Here's how the part is built. I have some questions about the finished solid (model axes, mm). Face numbers are marked on the shaded views. A direction names the side the tool comes from. Give positions to 0.01 mm unless a question says otherwise; leave off trailing zeros. Order: outer loops, then holes, each group sorted by start corner. A loop starts at its lowest first (then second) coordinate and runs counter-clockwise, first axis right, second up.
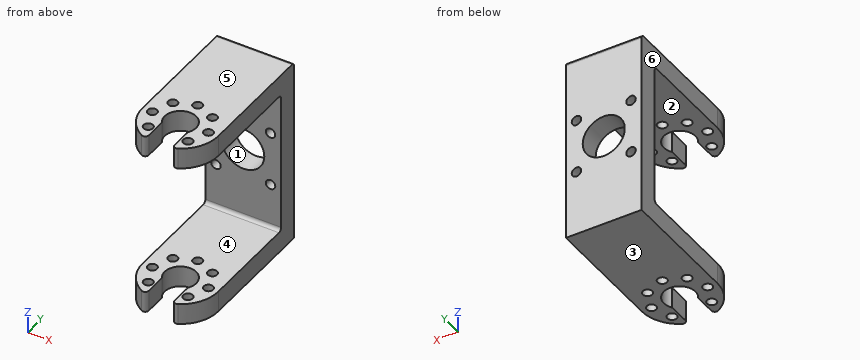
Autodesk Inventor part; units mm, degrees
ref_plane "YZ Plane" through (0, 0, 0) normal (1, 0, 0) x (0, 1, 0)
ref_plane "XZ Plane" through (0, 0, 0) normal (0, 1, 0) x (-1, 0, 0)
ref_plane "XY Plane" through (0, 0, 0) normal (0, 0, 1) x (1, 0, 0)
sketch "스케치1" plane through (0, 0, 0) normal (0, 0, 1) x (1, 0, 0)
  circle A0 centre (-22.9272, 17.0843) radius 10.8
  circle A1 centre (-22.9272, 17.0843) radius 6
  circle A2 centre (-22.9272, 9.0843) radius 1.05
  circle A3 centre (-28.584, 11.4274) radius 1.05
  circle A4 centre (-30.9272, 17.0843) radius 1.05
  circle A5 centre (-28.584, 22.7411) radius 1.05
  circle A6 centre (-22.9272, 25.0843) radius 1.05
  circle A7 centre (-17.2703, 22.7411) radius 1.05
  circle A8 centre (-14.9272, 17.0843) radius 1.05
  circle A9 centre (-17.2703, 11.4274) radius 1.05
  circle A10 centre (-28.584, 22.7411) radius 1.15
  circle A11 centre (-22.9272, 25.0843) radius 1.15
  circle A12 centre (-17.2703, 22.7411) radius 1.15
  circle A13 centre (-14.9272, 17.0843) radius 1.15
  circle A14 centre (-17.2703, 11.4274) radius 1.15
  circle A15 centre (-28.584, 11.4274) radius 1.15
  circle A16 centre (-30.9272, 17.0843) radius 1.15
  circle A17 centre (-22.9272, 17.0843) radius 3.5
  arc A18 (-19.2272, 17.0843) -> (-26.6272, 17.0843) centre (-22.9272, 17.0843) ccw
  arc A19 (-19.2272, 6.9378) -> (-26.6272, 6.9378) centre (-22.9272, 17.0843) ccw
  line L0 (-26.6272, 17.0843) -> (-26.6272, 6.9378)
  line L1 (-19.2272, 17.0843) -> (-19.2272, 6.9378)
  line L2 (-33.7272, 17.0843) -> (-33.7272, 52.0843)
  line L3 (-12.1272, 17.0843) -> (-12.1272, 52.0843)
  line L4 (-12.1272, 52.0843) -> (-33.7272, 52.0843)
  line L5 (-33.7272, 52.0843) -> (-12.1272, 52.0843)
  line L6 (-12.1272, 52.0843) -> (-12.1272, 58.0843)
  line L7 (-12.1272, 58.0843) -> (-33.7272, 58.0843)
  line L8 (-33.7272, 58.0843) -> (-33.7272, 52.0843)
  point P0 (0, 0)
  dimension "d0" = 0.1
  dimension "d1" = 0.1
  dimension "d2" = 0.1
  dimension "d3" = 0.1
  dimension "d4" = 0.1
  dimension "d5" = 0.1
  dimension "d6" = 0.1
  dimension "d7" = 0.2
  dimension "d8" = 35
  dimension "d9" = 35
  dimension "d10" = 6
extrude "돌출1" add sketch "스케치1" along normal blind 6 contours A0 L1 A1 L0 | A0 L2 L4 L3 | L1 A18 L0 A1 | A3 | A4 | A5 | A6 | A7 | A8 | A9 | A10 | A11 | A12 | A13 | A14 | A15 | A16 picked at (-19.6686, 25.2568) picked at (-26.9638, 14.2707)
sketch "스케치3" plane through (-33.7272, 52.0843, 0) normal (0, 1, 0) x (1, 0, 0)
  line L0 (0, -5.5) -> (21.6, -5.5)
  line L1 (21.6, -5.5) -> (21.6, 0.5)
  line L2 (0, -5.5) -> (0, 0.5)
  line L3 (0, -5.5) -> (21.6, -5.5)
  line L4 (0, -5.5) -> (21.6, -5.5)
  line L5 (21.6, -5.5) -> (21.6, 0.5)
  line L6 (0, -5.5) -> (0, 0.5)
  circle A0 centre (3.0218, -2.5) radius 1.45
  circle A1 centre (18.5782, -2.5) radius 1.45
  line L7 (21.6, 0.5) -> (21.6, 0)
  line L8 (21.6, 0) -> (0, 0)
  line L9 (0, 0) -> (0, 0.5)
  line L10 (21.6, 0) -> (0, 0)
  line L11 (0, 0) -> (0, -6)
  line L12 (21.6, -6) -> (0, -6)
  line L13 (21.6, 0) -> (21.6, -6)
  circle A2 centre (10.8, 20.55) radius 6
  line L14 (0, 0) -> (21.6, 0)
  line L15 (21.6, 0) -> (21.6, 41.1)
  line L16 (21.6, 41.1) -> (0, 41.1)
  line L17 (0, 41.1) -> (0, 0)
  line L18 (0, 41.1) -> (21.6, 41.1)
  line L19 (21.6, 41.1) -> (21.6, 47.1)
  line L20 (21.6, 47.1) -> (0, 47.1)
  line L21 (0, 47.1) -> (0, 41.1)
  circle A3 centre (18.5782, 12.7718) radius 1.35
  circle A4 centre (18.5782, 28.3282) radius 1.35
  circle A5 centre (3.0218, 28.3282) radius 1.35
  circle A6 centre (3.0218, 12.7718) radius 1.35
  point P0 (33.7272, 0)
  dimension "d13" = 2.9
  dimension "d14" = 2.9
  dimension "d19" = 0.5
  dimension "d24" = 12
  dimension "d25" = 41.1
  dimension "d26" = 6
  dimension "d29" = 2.7
  dimension "d30" = 2.7
  dimension "d31" = 2.7
  dimension "d32" = 2.7
extrude "돌출2" add sketch "스케치3" against normal blind 6 contours L2 L17 L16 L15 L1 L8
sketch "스케치5" plane through (-12.1272, 52.0843, -41.1) normal (0, 0, -1) x (-1, 0, 0)
  line L0 (19.9594, -6) -> (17.1969, -6)
  line L1 (17.1969, 0) -> (19.9594, 0)
  line L2 (4.4031, -6) -> (1.6406, -6)
  line L3 (1.6406, 0) -> (4.4031, 0)
  line L4 (4.4031, -6) -> (1.6406, -6)
  line L5 (1.6406, 0) -> (4.4031, 0)
  line L6 (0, 0) -> (0, -6)
  line L7 (0, 0) -> (21.6, 0)
  line L8 (0, 0) -> (0, -6)
  line L9 (21.6, -6) -> (0, -6)
  line L10 (21.6, 0) -> (21.6, -6)
  line L11 (0, 0) -> (21.6, 0)
  line L12 (21.6, -6) -> (0, -6)
  line L13 (21.6, 0) -> (21.6, -6)
  line L14 (19.9594, -6) -> (17.1969, -6)
  line L15 (17.1969, 0) -> (19.9594, 0)
  arc A0 (14.5, -35) -> (7.1, -35) centre (10.8, -35) ccw
  line L16 (16.8, -6) -> (4.8, -6)
  line L17 (16.8, -6) -> (4.8, -6)
  line L18 (4.8, 0) -> (16.8, 0)
  line L19 (4.8, 0) -> (16.8, 0)
  line L20 (21.6, -6) -> (0, -6)
  line L21 (21.6, -6) -> (0, -6)
  line L22 (16.8, -6) -> (4.8, -6)
  line L23 (4.8, 0) -> (16.8, 0)
  line L24 (0, 0) -> (21.6, 0)
  line L25 (0, 0) -> (21.6, 0)
  line L26 (21.6, -6) -> (21.6, -35)
  line L27 (21.6, 0) -> (21.6, -35)
  line L28 (21.6, 0) -> (21.6, -6)
  line L29 (0, -35) -> (0, -6)
  line L30 (0, 0) -> (0, -6)
  line L31 (0, -35) -> (0, 0)
  line L32 (1.6406, 0) -> (4.4031, 0)
  line L33 (4.4031, -6) -> (1.6406, -6)
  line L34 (1.6406, 0) -> (4.4031, 0)
  line L35 (17.1969, 0) -> (19.9594, 0)
  line L36 (19.9594, -6) -> (17.1969, -6)
  line L37 (17.1969, 0) -> (19.9594, 0)
  arc A1 (14.5, -35) -> (7.1, -35) centre (10.8, -35) ccw
  line L38 (0, -35) -> (0, -6)
  line L39 (0, 0) -> (21.6, 0)
  line L40 (0, -35) -> (0, 0)
  line L41 (19.9594, -6) -> (17.1969, -6)
  line L42 (21.6, -6) -> (0, -6)
  circle A2 centre (10.8, -12) radius 1.15
  circle A3 centre (5.1431, -14.3431) radius 1.15
  line L43 (21.6, 0) -> (21.6, -35)
  circle A4 centre (16.4569, -14.3431) radius 1.15
  circle A5 centre (10.8, -12) radius 1.15
  circle A6 centre (5.1431, -14.3431) radius 1.15
  line L44 (21.6, -6) -> (21.6, -35)
  circle A7 centre (16.4569, -14.3431) radius 1.15
  circle A8 centre (5.1431, -25.6569) radius 1.15
  circle A9 centre (5.1431, -25.6569) radius 1.15
  circle A10 centre (5.1431, -25.6569) radius 1.15
  circle A11 centre (5.1431, -25.6569) radius 1.15
  arc A12 (14.5, -45.1464) -> (21.6, -35) centre (10.8, -35) ccw
  arc A13 (14.5, -45.1464) -> (21.6, -35) centre (10.8, -35) ccw
  line L45 (14.5, -45.1464) -> (14.5, -35)
  line L46 (14.5, -45.1464) -> (14.5, -35)
  line L47 (7.1, -35) -> (7.1, -45.1464)
  line L48 (7.1, -35) -> (7.1, -45.1464)
  arc A14 (0, -35) -> (7.1, -45.1464) centre (10.8, -35) ccw
  arc A15 (0, -35) -> (7.1, -45.1464) centre (10.8, -35) ccw
  circle A16 centre (16.4569, -25.6569) radius 1.15
  circle A17 centre (16.4569, -25.6569) radius 1.15
  circle A18 centre (18.8, -20) radius 1.15
  circle A19 centre (18.8, -20) radius 1.15
  circle A20 centre (10.8, -12) radius 1.15
  circle A21 centre (10.8, -12) radius 1.15
  circle A22 centre (5.1431, -14.3431) radius 1.15
  circle A23 centre (5.1431, -14.3431) radius 1.15
  circle A24 centre (16.4569, -14.3431) radius 1.15
  circle A25 centre (16.4569, -14.3431) radius 1.15
  line L49 (21.6, -6) -> (0, -6)
  line L50 (0, -35) -> (0, -6)
  arc A26 (0, -35) -> (7.1, -45.1464) centre (10.8, -35) ccw
  line L51 (7.1, -35) -> (7.1, -45.1464)
  arc A27 (14.5, -35) -> (7.1, -35) centre (10.8, -35) ccw
  line L52 (14.5, -45.1464) -> (14.5, -35)
  arc A28 (14.5, -45.1464) -> (21.6, -35) centre (10.8, -35) ccw
  line L53 (21.6, -6) -> (21.6, -35)
  arc A29 (14.5, -45.1464) -> (21.6, -35) centre (10.8, -35) ccw
  line L54 (14.5, -45.1464) -> (14.5, -35)
  arc A30 (14.5, -35) -> (7.1, -35) centre (10.8, -35) ccw
  line L55 (7.1, -35) -> (7.1, -45.1464)
  arc A31 (0, -35) -> (7.1, -45.1464) centre (10.8, -35) ccw
  line L56 (0, -35) -> (0, 0)
  line L57 (0, 0) -> (21.6, 0)
  line L58 (21.6, 0) -> (21.6, -35)
  arc A32 (14.5, -35) -> (7.1, -35) centre (10.8, -35) ccw
  arc A33 (14.5, -35) -> (7.1, -35) centre (10.8, -35) ccw
  circle A34 centre (2.8, -20) radius 1.15
  circle A35 centre (2.8, -20) radius 1.15
  circle A36 centre (18.8, -20) radius 1.15
  circle A37 centre (18.8, -20) radius 1.15
  arc A38 (0, -35) -> (7.1, -45.1464) centre (10.8, -35) ccw
  arc A39 (0, -35) -> (7.1, -45.1464) centre (10.8, -35) ccw
  line L59 (7.1, -35) -> (7.1, -45.1464)
  line L60 (7.1, -35) -> (7.1, -45.1464)
  arc A40 (14.5, -45.1464) -> (21.6, -35) centre (10.8, -35) ccw
  arc A41 (14.5, -45.1464) -> (21.6, -35) centre (10.8, -35) ccw
  line L61 (14.5, -45.1464) -> (14.5, -35)
  line L62 (14.5, -45.1464) -> (14.5, -35)
  circle A42 centre (16.4569, -25.6569) radius 1.15
  circle A43 centre (16.4569, -25.6569) radius 1.15
  line L63 (4.4031, -6) -> (1.6406, -6)
  circle A44 centre (2.8, -20) radius 1.05
  circle A45 centre (5.1431, -25.6569) radius 1.05
  circle A46 centre (5.1431, -14.3431) radius 1.05
  circle A47 centre (10.8, -12) radius 1.05
  circle A48 centre (16.4569, -14.3431) radius 1.05
  circle A49 centre (18.8, -20) radius 1.05
  circle A50 centre (16.4569, -25.6569) radius 1.05
  point P0 (-12.1272, -52.0843)
  point P1 (21.6, -6)
  point P2 (0, -6)
  point P3 (21.6, -6)
  point P4 (0, -6)
  point P5 (0, -6)
  dimension "d34" = 0.1
  dimension "d35" = 0.1
  dimension "d36" = 0.1
  dimension "d37" = 0.1
  dimension "d38" = 0.1
  dimension "d39" = 0.1
extrude "돌출4" add sketch "스케치5" along normal blind 6 contours L9 L26 A12 L45 A0 L47 A14 L29 L2 L0 | L0 L9 L2 L6 L7 L3 L1 L10 | A2 | A3 | A4 | A8 | A16 | A18 | A34 | A44 | A45 | A46 | A47 | A48 | A49 | A50
sketch "스케치6" plane through (0, 0, 6) normal (0, 0, 1) x (1, 0, 0)
  arc A0 (-33.7272, 17.0843) -> (-26.6272, 6.9378) centre (-22.9272, 17.0843) ccw
  line L0 (-26.6272, 6.9378) -> (-26.6272, 17.0843)
  arc A1 (-19.2272, 17.0843) -> (-26.6272, 17.0843) centre (-22.9272, 17.0843) ccw
  line L1 (-19.2272, 17.0843) -> (-19.2272, 6.9378)
  arc A2 (-19.2272, 6.9378) -> (-12.1272, 17.0843) centre (-22.9272, 17.0843) ccw
  line L2 (-12.1272, 17.0843) -> (-12.1272, 52.0843)
  line L3 (-12.1272, 52.0843) -> (-33.7272, 52.0843)
  line L4 (-33.7272, 52.0843) -> (-33.7272, 17.0843)
  circle A3 centre (-17.2703, 22.7411) radius 1.05
  circle A4 centre (-22.9272, 25.0843) radius 1.05
  circle A5 centre (-28.584, 22.7411) radius 1.05
  circle A6 centre (-30.9272, 17.0843) radius 1.05
  circle A7 centre (-28.584, 11.4274) radius 1.05
  circle A8 centre (-17.2703, 11.4274) radius 1.05
  circle A9 centre (-14.9272, 17.0843) radius 1.05
  circle A10 centre (-28.584, 22.7411) radius 1.35
  circle A11 centre (-22.9272, 25.0843) radius 1.35
  circle A12 centre (-17.2703, 22.7411) radius 1.35
  circle A13 centre (-14.9272, 17.0843) radius 1.35
  circle A14 centre (-17.2703, 11.4274) radius 1.35
  circle A15 centre (-28.584, 11.4274) radius 1.35
  circle A16 centre (-30.9272, 17.0843) radius 1.35
  point P0 (0, 0)
  dimension "d40" = 2.7
  dimension "d41" = 2.7
  dimension "d42" = 2.7
  dimension "d43" = 2.7
  dimension "d44" = 2.7
  dimension "d45" = 2.7
  dimension "d46" = 2.7
extrude "돌출5" cut sketch "스케치6" against normal blind 100 contours A3 | A4 | A5 | A6 | A7 | A8 | A9 | A10 | A11 | A12 | A13 | A14 | A15 | A16
fillet "모깎기2" radius 1 7 edges at (-26.6272, 6.9378, 3) (-26.6272, 6.9378, -44.1) (-19.2272, 6.9378, 3) (-19.2272, 6.9378, -44.1) (-22.9272, 46.0843, -41.1) (-22.9272, 46.0843, 0) (-22.9272, 52.0843, 6)
sketch "스케치7" plane through (-12.1272, 52.0843, -47.1) normal (0, 0, -1) x (-1, 0, 0)
  circle A0 centre (16.4569, -29.3431) radius 1.35
  circle A1 centre (18.8, -35) radius 1.35
  circle A2 centre (5.1431, -40.6569) radius 1.35
  circle A3 centre (10.8, -27) radius 1.35
  circle A4 centre (5.1431, -29.3431) radius 1.35
  circle A5 centre (16.4569, -40.6569) radius 1.35
  circle A6 centre (2.8, -35) radius 1.35
  line L0 (0, -1) -> (21.6, -1)
  line L1 (0, -1) -> (0, -35)
  arc A7 (0, -35) -> (5.6204, -44.4769) centre (10.8, -35) ccw
  arc A8 (5.6204, -44.4769) -> (7.1, -43.5994) centre (6.1, -43.5994) ccw
  line L2 (7.1, -43.5994) -> (7.1, -35)
  arc A9 (14.5, -35) -> (7.1, -35) centre (10.8, -35) ccw
  line L3 (14.5, -35) -> (14.5, -43.5994)
  arc A10 (14.5, -43.5994) -> (15.9796, -44.4769) centre (15.5, -43.5994) ccw
  arc A11 (15.9796, -44.4769) -> (21.6, -35) centre (10.8, -35) ccw
  line L4 (21.6, -35) -> (21.6, -1)
  circle A12 centre (10.8, -35) radius 4.5
  point P0 (-12.1272, -52.0843)
  dimension "d51" = 9
extrude "돌출6" cut sketch "스케치7" against normal blind 100 contours A12 L3 A9 L2 | L2 A9 L3 A12
properties part number "3D_upper_to_arm1" material "PMMA 플라스틱"
Q1. I need wall thicknesses on L1, parallel to Z at x = -29, y = 26; L2, parallel to X at y = 11, z = 1.5; L3, parallel to Z at x = -27.75, y = 47. Which ranges of each line are inside material? Lowest first, please.
Filled sheet:
L1: z = -47.1 to -41.1, 0 to 6
L2: x = -31.85 to -29.86, -27.3 to -26.63, -19.23 to -18.55, -15.99 to -14
L3: z = -47.1 to -24.12, -16.98 to 6
Q2. I'm going to push flat-ended pins straight in: P1, Ø8, axis at x = -19, z = -17, coming from the -Y side; P2, Ø5, axis at y = 11.5, z = -44, coming from the +X side; P3, Ø1.8, axis at y = 11, z = 3.5, coming from the +X side. Where does each tip first touch, or does it pass through?
Filled sheet:
P1: stops at y = 46.08
P2: stops at x = -12.58
P3: stops at x = -13.45
Q3. If we section it at C-C on x = -22.5: List the corners of the cut face in (y, z) for me, plus the area to 3 significant figures.
Filled sheet:
outline: (21.56, -47.1) - (23.8, -47.1) - (23.8, -41.1) - (21.56, -41.1) - close; (21.56, 0) - (23.8, 0) - (23.8, 6) - (21.56, 6) - close; (26.36, -47.1) - (52.08, -47.1) - (52.08, -26.53) - (46.08, -26.53) - (46.08, -40.1) arc R1 cw to (45.08, -41.1) - (26.36, -41.1) - close; (26.36, 0) - (45.08, 0) arc R1 cw to (46.08, -1) - (46.08, -14.57) - (52.08, -14.57) - (52.08, 5) arc R1 ccw to (51.08, 6) - (26.36, 6) - close
area: 511 mm2
Q4. Thinking about a two-plate mould opening in Z: for the marked faces 3, 4, 5 and 6, which applies, released by +Z, released by -Z, zero draft, split by the parting line, or undercut?
Filled sheet:
face 3: released by -Z
face 4: undercut
face 5: released by +Z
face 6: zero draft
Q5. For the marked faces 1 and 2, which set-ups out of +Z, -Z, +X, -X, +Y, -Y let a thin tool reach every point of the face, with its end or its side?
Filled sheet:
face 1: +Y, -Y
face 2: +X, -X, -Y
Q6. If we section it at B-B on y = 41: List the corners of the cut face in (x, z) for me.
Filled sheet:
outline: (-33.73, -47.1) - (-12.13, -47.1) - (-12.13, -41.1) - (-33.73, -41.1) - close; (-33.73, 0) - (-12.13, 0) - (-12.13, 6) - (-33.73, 6) - close
Q7. If we section it at A-A on z = -20.55: List the corners of the cut face in (x, y) for me, plus the area to 3 significant figures.
Filled sheet:
outline: (-33.73, 46.08) - (-28.93, 46.08) - (-28.93, 52.08) - (-33.73, 52.08) - close; (-16.93, 46.08) - (-12.13, 46.08) - (-12.13, 52.08) - (-16.93, 52.08) - close
area: 57.6 mm2
Q8. If we section it at D-D on x = -15: List the corners of the cut face in (y, z) for me.
Filled sheet:
outline: (9.75, -47.1) - (15.74, -47.1) - (15.74, -41.1) - (9.75, -41.1) - close; (9.75, 0) - (15.74, 0) - (15.74, 6) - (9.75, 6) - close; (18.43, -47.1) - (52.08, -47.1) - (52.08, -29.67) - (46.08, -29.67) - (46.08, -40.1) arc R1 cw to (45.08, -41.1) - (18.43, -41.1) - close; (18.43, 0) - (45.08, 0) arc R1 cw to (46.08, -1) - (46.08, -11.43) - (52.08, -11.43) - (52.08, 5) arc R1 ccw to (51.08, 6) - (18.43, 6) - close; (46.08, -26.99) - (52.08, -26.99) - (52.08, -14.11) - (46.08, -14.11) - close
